```python
from build123d import *

# Parameters (mm, degrees)
SKETCH2_R                = 50
BOSS_EXTRUDE1_DEPTH      = 5
SKETCH3_W                = 60
SKETCH3_H                = 60
BOSS_EXTRUDE2_DEPTH      = 60
CUT_EXTRUDE14_DEPTH      = 150
CUT_EXTRUDE15_DEPTH      = 150
CUT_EXTRUDE16_DEPTH      = 71
CUT_EXTRUDE16_DEPTH_BACK = 56
SKETCH31_R               = 10
BOSS_EXTRUDE5_DEPTH      = 5
BOSS_EXTRUDE6_START      = 5
SKETCH32_R               = 10
BOSS_EXTRUDE6_DEPTH      = 5


with BuildPart() as part:
    # Sketch2 → Boss-Extrude1 (new body)
    with BuildSketch(Plane(origin=(0, 0, 0), x_dir=(1, 0, 0), z_dir=(0, 1, 0))):
        with Locations(Location((0, 0, 0), (0, 0, 270))):
            Circle(SKETCH2_R)
    extrude(amount=BOSS_EXTRUDE1_DEPTH)

    # Sketch3 → Boss-Extrude2 (add)
    with BuildSketch(Plane(origin=(0, 5, 0), x_dir=(1, 0, 0), z_dir=(0, 1, 0))):
        Rectangle(SKETCH3_W, SKETCH3_H)
    extrude(amount=BOSS_EXTRUDE2_DEPTH)

    # Sketch19 → Cut-Extrude14 (cut)
    with BuildSketch(Plane.XY.offset(30)):
        with BuildLine():
            Line((-10, 5), (-10, 55))
            ThreePointArc((-10, 55), (-7.071067812, 62.071067812), (0, 65))
            Line((0, 65), (-30, 65))
            Line((-30, 65), (-30, 5))
            Line((-30, 5), (-10, 5))
        make_face()
    extrude(amount=-CUT_EXTRUDE14_DEPTH, mode=Mode.SUBTRACT)

    # Sketch29 → Cut-Extrude15 (cut)
    with BuildSketch(Plane.XY.offset(30)):
        with BuildLine():
            Line((30, 65), (0, 65))
            ThreePointArc((0, 65), (7.071067812, 62.071067812), (10, 55))
            Line((10, 55), (10, 5))
            Line((10, 5), (30, 5))
            Line((30, 5), (30, 65))
        make_face()
    extrude(amount=-CUT_EXTRUDE15_DEPTH, mode=Mode.SUBTRACT)

    # Sketch30 → Cut-Extrude16 (cut, two sides: drawn at the far end of the back side and taken through both)
    with BuildSketch(Plane(origin=(0, 0, 0), x_dir=(0, 0, -1), z_dir=(1, 0, 0)).offset(-CUT_EXTRUDE16_DEPTH_BACK)):
        with BuildLine():
            Line((20, 65), (-20, 65))
            Line((-20, 65), (-20, 55))
            add(Edge.make_bspline(
                [(-20, 55), (-21.218129455, 29.129128635), (-9.16621621, 5)],
                knots=[0, 0, 0, 1, 1, 1], degree=2))
            Line((-9.16621621, 5), (9.16621621, 5))
            add(Edge.make_bspline(
                [(20, 55), (21.218129455, 29.129128635), (9.16621621, 5)],
                knots=[0, 0, 0, 1, 1, 1], degree=2))
            Line((20, 55), (20, 65))
        make_face()
    extrude(amount=CUT_EXTRUDE16_DEPTH + CUT_EXTRUDE16_DEPTH_BACK, mode=Mode.SUBTRACT)

    # Sketch31 → Boss-Extrude5 (add)
    with BuildSketch(Plane(origin=(0, 0, 20), x_dir=(-1, 0, 0), z_dir=(0, 0, -1))):
        with Locations(Location((0, 55, 0), (0, 0, 180))):
            Circle(SKETCH31_R)
    extrude(amount=BOSS_EXTRUDE5_DEPTH)

    # Sketch32 → Boss-Extrude6 (add)
    with BuildSketch(Plane.XY.offset(-20).offset(BOSS_EXTRUDE6_START)):
        with Locations((0, 55)):
            Circle(SKETCH32_R)
    extrude(amount=-BOSS_EXTRUDE6_DEPTH)


solid = part.part
```
For this review, take the finished solid that the model builds, in its own axes (mm). A direction names the side the tool comes from. Round coordinates to 2 decimals unless told otherwise and drop trailing zeros. Write each loop counter-clockwise with the first axis right and the second up, starting at its lowest first coordinate (ties: lowest second). Pieces come first, ordered by that corner, then holes. Notation, with made-up numbers: (-23.5, -36) -> (5.5, -36) arc R20 cw to (5.5, -3) -> close; hole circle Ø1 at (-10.75, 63). An arc over 180 degrees is marked (long way). Use one line per item in the form item = value.
1) Take a section at C-C, the plane x = -40. Write out the cut boundary in (y, z), and give its area (3 significant figures).
Found:
outline = (0, -30) -> (5, -30) -> (5, 30) -> (0, 30) -> close
area = 300 mm2
2) Clearance check with flat-ended pins moving along their axes: pin 1 (6 mm diameter, centred on x = -4.5, y = 42, fed in from -Z); pin 2 (4.5 mm diameter, centred on x = 3.5, y = 49.5, fed in from +Z); pin 3 (23 mm diameter, centred on y = 24, z = 24, fed in from +X); pin 4 (12 mm diameter, centred on x = -23.5, y = 14.5, fed in from +Z). State where each tip first meets the part, or that it passes through.
Found:
pin_1 = -30
pin_2 = 30
pin_3 = 10
pin_4 = through
3) Take a section at A-A, the plane z = 27. Write out the cut boundary in (x, y).
Found:
outline = (-42.08, 0) -> (42.08, 0) -> (42.08, 5) -> (10, 5) -> (10, 55) arc R10 ccw to (-10, 55) -> (-10, 5) -> (-42.08, 5) -> close
4) Take a section at B-B, the plane y = 50. Count the separate pieces of the cut face and the enclosed holes in it, and give its area (3 significant figures).
Found:
separate_pieces = 4
enclosed_holes = 0
area = 569 mm2
5) Tool access review of faces 1 (the flat face through (-10, 24, -24)), 2 (the flat face through (0, 55, 15)), 3 (the flat face through (0, 35, -30)), 4 (the flat face through (0, 35, 30)): name each direction out of +Z, -Z, +X, -X, +Y, -Y from which nothing blocks a thin tool from reaching the whole face with its end or side.
Found:
face_1 = +Z, -Z, -X, +Y
face_2 = +X, -X, +Y
face_3 = -Z, +X, -X, +Y
face_4 = +Z, +X, -X, +Y
6) Take a section at D-D, the plane z = 0. Write out the cut boundary in (x, y), and give its area (3 significant figures).
Found:
outline = (-50, 0) -> (50, 0) -> (50, 5) -> (-50, 5) -> close
area = 500 mm2
7) Mouldability with a two-part tool opening along Z and no side actions: class faces 5 (the cylindrical face through (15.02, 2.46, 47.69)), 6 (the flat face through (0, 55, -15)), 7 (the flat face through (10, 25, -24)) as +Z half, -Z half, draft (parallel to the pull), parting line (faces both ways), or undercut.
Found:
face_5 = parting line
face_6 = undercut
face_7 = draft
8) To check wall thickness, follow L1, parallel to Y at x = 37, z = -24; L2, parallel to Z at x = 5, y = 10.5; L3, parallel to Z at x = -7, y = 36.5. State the ranges of each line that lie inside material, in increasing order. Write a range as from..to.
Found:
L1 = 0..5
L2 = -30..-11.73, 11.73..30
L3 = -30..-19.14, 19.14..30
